Design review of the part shown in the three views and the two pictorial views. Dimensions are in mm from the part's minimum x, y and z. A direction names the side the tool comes from. Round coordinates to 2 decimals unless told otherwise and drop trailing zeros. Order: outer loops, then holes, each group sorted by start corner. A loop starts at its lowest first (then second) coordinate and runs counter-clockwise, first axis right, second up. Notation, with made-up numbers: (23, -21.5) -> (75, -21.5) arc R17 ccw to (75, 8.5) -> close; hole circle Ø7 at (86.5, 89.25). An arc over 180 degrees is marked (long way). Put each result on its own line as item: value. Start each with the question number.
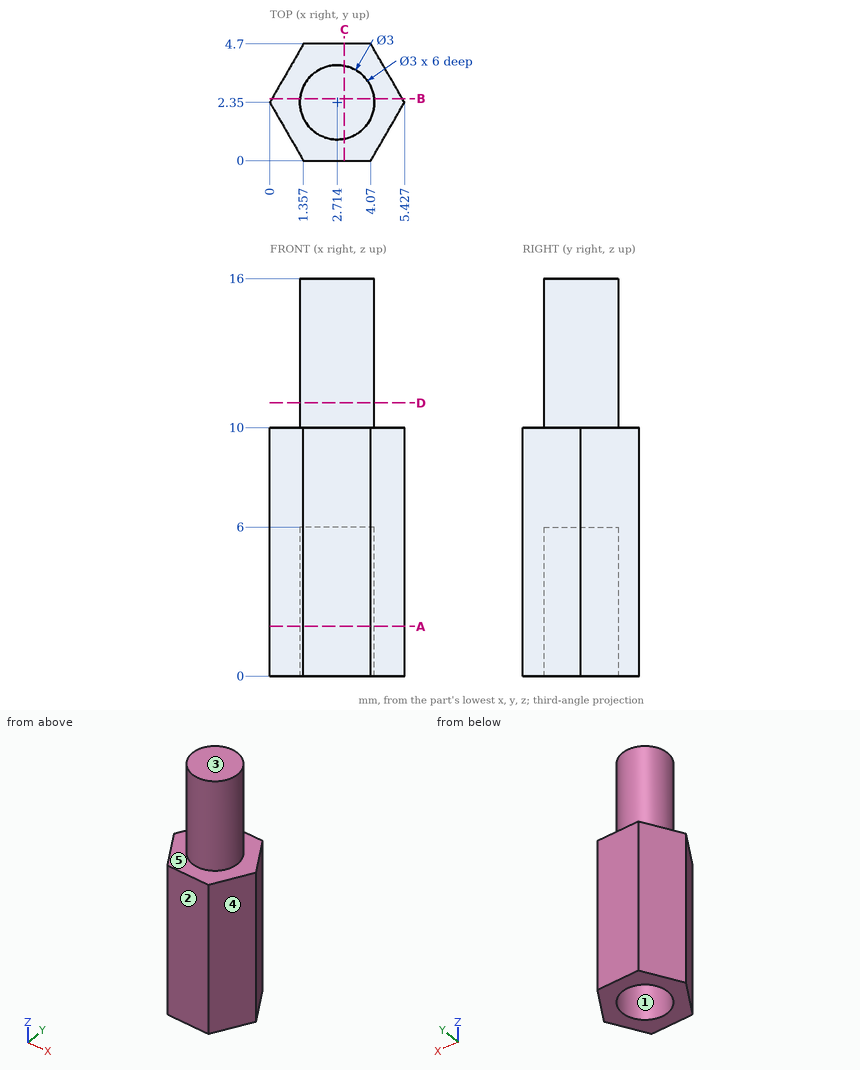
Q1. Wall thickness on probe 1 along Z at (x, y) = (1, 3.5); probe 2 along Z at (x, y) = (1.9, 2.9); probe 3 along Y at (x, z) = (2.35, 5.5) (1 decimal): over which ranges is each line inside the solid? List them lowest first. Write a range as [from, to].
Q2. Take a section at A-A on z = 2. Give the boundary of the cut face in (x, y).
Q3. Take a section at C-C on x = 3. Give the boundary of the cut face in (y, z), and give its area (3 significant figures).
Q4. Clearance check with a flat-ended pin moving along its axis: pin 1 Ø1 at (x, y) = (2.5, 2) entering from -Z. State where the tip first meets the part, or that it passes through.
Q5. For the marked faces 4 and 5, list the 3-axis set-ups (+Z, -Z, +X, -X, +Y, -Y) from which the entire face can be reached by the end or side of a thin tool; tool diameter is ignored.
Q6. Take a section at D-D on z = 11. Give the boundary of the cut face in (x, y).
Q7. Draft analysis for pull direction Y (two halves, no side actions). For the marked faces 1, 2 and 3, state which applies: +Y half, -Y half, draft (parallel to the pull), parting line (faces both ways), or undercut.
Q8. Take a section at B-B on y = 2.5. Give the boundary of the cut face in (x, z).
Calculated:
1. probe 1: z = [0, 10]
1. probe 2: z = [6, 16]
1. probe 3: y = [0, 0.9], [3.8, 4.7]
2. outline: (0, 2.35) -> (1.36, 0) -> (4.07, 0) -> (5.43, 2.35) -> (4.07, 4.7) -> (1.36, 4.7) -> close; hole circle Ø3 at (2.71, 2.35)
3. outline: (0, 0) -> (0.88, 0) -> (0.88, 6) -> (3.82, 6) -> (3.82, 0) -> (4.7, 0) -> (4.7, 10) -> (3.82, 10) -> (3.82, 16) -> (0.88, 16) -> (0.88, 10) -> (0, 10) -> close
3. area: 47.0 mm²
4. pin 1: stops at z = 6
5. face 4: +Z, -Z, +X, -Y
5. face 5: +Z
6. outline: circle Ø3 at (2.71, 2.35)
7. face 1: undercut
7. face 2: -Y half
7. face 3: draft
8. outline: (0.09, 0) -> (1.22, 0) -> (1.22, 6) -> (4.21, 6) -> (4.21, 0) -> (5.34, 0) -> (5.34, 10) -> (4.21, 10) -> (4.21, 16) -> (1.22, 16) -> (1.22, 10) -> (0.09, 10) -> close
